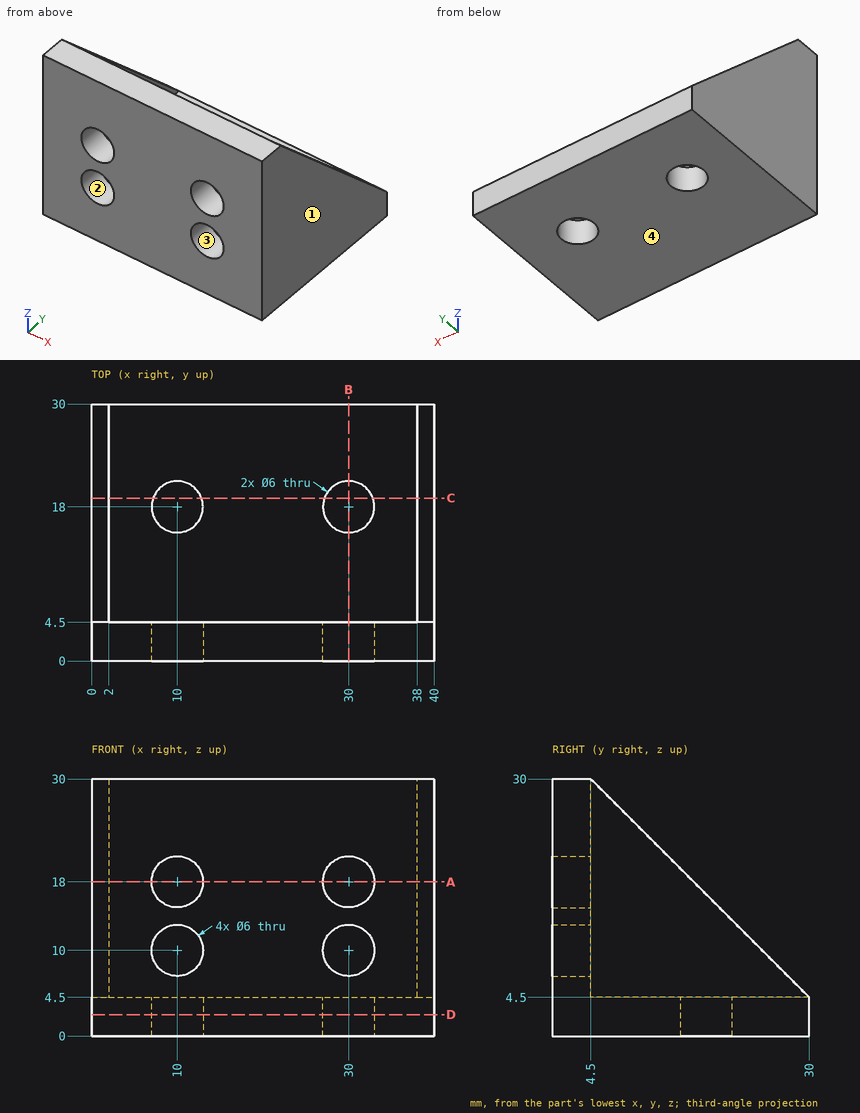
Answer from the drawing. Dimensions are ordinates in mm from the lowest x, y and z of the part. Give positions to 0.01 mm unless a question says otherwise; leave off trailing zeros. Write each loop counter-clockwise with the first axis right and the second up, starting at its lowest first coordinate (ties: lowest second). Pieces come first, ordered by that corner, then holes. Notation, with made-up numbers: (-36, 65.5) - (17, 65.5) arc R26 cw to (17, 93.5) - close; hole circle Ø2 at (-26.5, -40). An arc over 180 degrees is marked (long way). Answer in a Markdown table with one row per item. Add a question column.
Item 1: Section A-A, the plane z = 18 is taken. Write down the section's boundary in (x, y).
Item 2: Section C-C, the plane y = 19 is taken. Write down the section's boundary in (x, z), and give its area (3 significant figures).
Item 3: Find the intervals of material crossed by L1, parallel to X at y = 1.65, z = 18; L2, parallel to Z at x = 30, y = 1.95; L3, parallel to Y at x = 30, z = 2.9, in increasing order.
Item 4: Flat-ended cylindrical pins translate along their axes: P1, Ø3, axis at x = 22, z = 14.5, coming from the -Y side; P2, Ø5, axis at x = 25, y = 10, coming from the +Z side; P3, Ø5.5, axis at x = 10, z = 18, coming from the +Y side; P4, Ø12, axis at x = 8.5, z = 14, coming from the +Y side. Find the tip coordinate at first contact, or state that the pin passes through.
Item 5: Section B-B, the plane x = 30 is taken. Write down the section's boundary in (y, z).
Item 6: Section D-D, the plane z = 2.5 is taken. Write down the section's boundary in (x, y).
Item 7: Determine the mould class of the marked faces 1, 2, 3 and 4 for opening direction Z: pulls with the +Z half, pulls with the -Z half, needs draft (parallel to the pull), parting line crosses it, or undercut.
Recorded:
| question | item | result |
|---|---|---|
| 1 | outline | (0, 0) - (7, 0) - (7, 4.5) - (2, 4.5) - (2, 16.5) - (0, 16.5) - close; (13, 0) - (27, 0) - (27, 4.5) - (13, 4.5) - close; (33, 0) - (40, 0) - (40, 16.5) - (38, 16.5) - (38, 4.5) - (33, 4.5) - close |
| 2 | outline | (0, 0) - (7.17, 0) - (7.17, 4.5) - (2, 4.5) - (2, 15.5) - (0, 15.5) - close; (12.83, 0) - (27.17, 0) - (27.17, 4.5) - (12.83, 4.5) - close; (32.83, 0) - (40, 0) - (40, 15.5) - (38, 15.5) - (38, 4.5) - (32.83, 4.5) - close |
| 2 | area | 173 mm2 |
| 3 | L1 | x = 0 to 7, 13 to 27, 33 to 40 |
| 3 | L2 | z = 0 to 7, 13 to 15, 21 to 30 |
| 3 | L3 | y = 0 to 15, 21 to 30 |
| 4 | P1 | stops at y = 0 |
| 4 | P2 | stops at z = 4.5 |
| 4 | P3 | passes through |
| 4 | P4 | stops at y = 4.5 |
| 5 | outline | (0, 0) - (15, 0) - (15, 4.5) - (4.5, 4.5) - (4.5, 7) - (0, 7) - close; (0, 13) - (4.5, 13) - (4.5, 15) - (0, 15) - close; (0, 21) - (4.5, 21) - (4.5, 30) - (0, 30) - close; (21, 0) - (30, 0) - (30, 4.5) - (21, 4.5) - close |
| 6 | outline | (0, 0) - (40, 0) - (40, 30) - (0, 30) - close; hole circle Ø6 at (10, 18); hole circle Ø6 at (30, 18) |
| 7 | face 1 | needs draft |
| 7 | face 2 | undercut |
| 7 | face 3 | undercut |
| 7 | face 4 | pulls with the -Z half |
